Input: part model. Units: mm. Frame: model coordinates. A direction names the side the tool comes from. Coordinates: 2 decimals unless noted, no trailing zeros. Write each loop counter-clockwise with the first axis right and the second up, starting at its lowest first coordinate (ties: lowest second). Pieces come first, ordered by that corner, then holes. Notation, with made-up numbers: M -23.75,11 L -5.75,11 A34 ccw -5.75,50 Z; hole C 7,1.25 d3. An arc over 180 degrees is marked long. Write each question's results on one line, items separated by ' | '. Start each with the question number.
1. Section query B-B, the plane x = 0. Output: boundary loops of the cut face in (y, z), and give its area (3 significant figures).
2. Section query A-A, the plane z = 0. Output: boundary loops of the cut face in (x, y).
3. Ray query, probe 1 along Y at (x, z) = (4.5, 5.5); probe 2 along Y at (x, z) = (1.25, -1.25); probe 3 along X at (y, z) = (-18.75, -0.25). Return the intervals inside material, ascending.
4. Section query C-C, the plane y = -22.25. Output: boundary loops of the cut face in (x, z).
5. Pull-direction query (Z, two-part tool) for faces 3 (the flat face through (0, -29, 0)), 4 (the flat face through (0, -9, 7.599)), 5 (the cylindrical face through (-10, -9, 0)); classes: +Z half, -Z half, draft (parallel to the pull), parting line (faces both ways), or undercut.
6. Section query D-D, the plane z = -2.5. Output: boundary loops of the cut face in (x, y), and give its area (3 significant figures).
7. First-contact query: pin 1 (2 mm diameter, centred on y = -12.5, z = 3, fed in from -X); pin 2 (3 mm diameter, centred on y = -5.5, z = 3.5, fed in from +X); pin 3 (6 mm diameter, centred on y = -15.5, z = 5.5, fed in from +X). Flat tips, straight axial feed; report the tip coordinate or a pass-through.
8. Set-up query: faces 1 (the cylindrical face through (-3, -20, 0)), 2 (the flat face through (0, 0, 0)). Return all of +Z, -Z, +X, -X, +Y, -Y with unobstructed straight access to the full face (end or side cutting, diameter ignored); none if empty.
```python
from build123d import *

# Parameters (mm, degrees)
F1_DEPTH = 19
F2_R     = 3
F3_DEPTH = 1.5
F4_R     = 1
F5_DEPTH = 8.5


with BuildPart() as f1:
    # F0 (on Front) → F1 (new body)
    with BuildSketch(Plane.XZ):
        with BuildLine():
            Line((6.5, 7.599342), (-6.5, 7.599342))
            ThreePointArc((-6.5, 7.599342), (-10, 0), (-6.5, -7.599342))
            Line((-6.5, -7.599342), (6.5, -7.599342))
            ThreePointArc((6.5, -7.599342), (10, 0), (6.5, 7.599342))
        make_face()
    extrude(amount=F1_DEPTH)

    # F2 (on face) → F3 (join)
    with BuildSketch(Plane.XZ.offset(19)):
        Circle(F2_R)
    extrude(amount=F3_DEPTH)

    # F4 (on face) → F5 (join)
    with BuildSketch(Plane.XZ.offset(20.5)):
        Circle(F4_R)
    extrude(amount=F5_DEPTH)


solid = f1.part
```
Answer:
1) outline: M -29,-1 L -20.5,-1 L -20.5,-3 L -19,-3 L -19,-7.6 L 0,-7.6 L 0,7.6 L -19,7.6 L -19,3 L -20.5,3 L -20.5,1 L -29,1 Z | area: 315 mm^2
2) outline: M -10,-19 L -3,-19 L -3,-20.5 L -1,-20.5 L -1,-29 L 1,-29 L 1,-20.5 L 3,-20.5 L 3,-19 L 10,-19 L 10,0 L -10,0 Z
3) probe 1: -19 to 0 | probe 2: -20.5 to 0 | probe 3: -10 to 10
4) outline: C 0,0 d2
5) face 3: draft | face 4: +Z half | face 5: parting line
6) outline: M -9.68,-19 L -1.66,-19 L -1.66,-20.5 L 1.66,-20.5 L 1.66,-19 L 9.68,-19 L 9.68,0 L -9.68,0 Z | area: 373 mm^2
7) pin 1: x = -9.8 | pin 2: x = 9.8 | pin 3: x = 9.68
8) face 1: -Y | face 2: +Z, -Z, +X, -X, +Y
